from build123d import *

# Parameters (mm, degrees)
SKETCH1_W           = 44.45
SKETCH1_H           = 19.05
SKETCH1_W_2         = 38.1
SKETCH1_H_2         = 12.7
BOSS_EXTRUDE1_DEPTH = 12.7
CUT_EXTRUDE1_REACH  = 33.908
SKETCH2_R           = 2.0955
SKETCH3_W           = 50.8
SKETCH3_H           = 25.4
BOSS_EXTRUDE2_DEPTH = 3.175


with BuildPart() as part:
    # Sketch1 → Boss-Extrude1 (new body)
    with BuildSketch(Plane.XY):
        Rectangle(SKETCH1_W, SKETCH1_H)
        Rectangle(SKETCH1_W_2, SKETCH1_H_2, mode=Mode.SUBTRACT)
    extrude(amount=BOSS_EXTRUDE1_DEPTH)

    # Cut-Extrude1: up to this face of the body (flat: up to its plane)
    cut_extrude1_end = Plane(part.part.faces().sort_by_distance((0, -9.525, 6.35))[0])
    # Sketch2 → Cut-Extrude1 (cut, up to the picked face)
    with BuildSketch(Plane(origin=(0, 9.525, 0), x_dir=(1, 0, 0), z_dir=(0, 1, 0)), mode=Mode.PRIVATE) as cut_extrude1_sk1:
        with Locations(Location((-12.7, -6.35, 0), (0, 0, 270))):
            Circle(SKETCH2_R)
    cut_extrude1_tool1 = split(extrude(cut_extrude1_sk1.sketch, amount=-CUT_EXTRUDE1_REACH, mode=Mode.PRIVATE), bisect_by=cut_extrude1_end, keep=Keep.BOTH, mode=Mode.PRIVATE)
    # Sketch2 → Cut-Extrude1 (cut, up to the picked face)
    with BuildSketch(Plane(origin=(0, 9.525, 0), x_dir=(1, 0, 0), z_dir=(0, 1, 0)), mode=Mode.PRIVATE) as cut_extrude1_sk2:
        with Locations(Location((12.7, -6.35, 0), (0, 0, 90))):
            Circle(SKETCH2_R)
    cut_extrude1_tool2 = split(extrude(cut_extrude1_sk2.sketch, amount=-CUT_EXTRUDE1_REACH, mode=Mode.PRIVATE), bisect_by=cut_extrude1_end, keep=Keep.BOTH, mode=Mode.PRIVATE)
    add(cut_extrude1_tool1.solids().sort_by(Axis((-12.7, 9.525, 6.35), (0, -1, 0)))[0], mode=Mode.SUBTRACT)
    add(cut_extrude1_tool2.solids().sort_by(Axis((12.7, 9.525, 6.35), (0, -1, 0)))[0], mode=Mode.SUBTRACT)

    # Sketch3 → Boss-Extrude2 (add)
    with BuildSketch(Plane(origin=(0, 0, 0), x_dir=(-1, 0, 0), z_dir=(0, 0, -1))):
        Rectangle(SKETCH3_W, SKETCH3_H)
    extrude(amount=BOSS_EXTRUDE2_DEPTH)


solid = part.part
Build history of the part. All positions in model axes, mm. A direction names the side the tool comes from. Coordinates: 2 decimals unless noted, no trailing zeros. Write each loop counter-clockwise with the first axis right and the second up, starting at its lowest first coordinate (ties: lowest second). Pieces come first, ordered by that corner, then holes.
(1) Cut at A-A on x = 12.7. State how many separate pieces and enclosed holes the cut face has, and give its area (3 significant figures).
(2) Mould opens along Z. For faces 4 (the flat face through (-0.3, 6.5, 12.7)), 5 (the cylindrical face through (-10.62, -7.92, 6.08)), 6 (the flat face through (0, 0, -3.175)) say: pulls with the +Z half, pulls with the -Z half, needs draft (parallel to the pull), parting line crosses it, or undercut.
(3) Cut at D-D on x = -7. List the corners of the cut face in (y, z) (3 decimals), and give its area (3 significant figures).
(4) Cut at C-C on y = 2.5. List the corners of the cut face in (x, z) (3 decimals), and give its area (3 significant figures).
(5) Drill centre lines: line 1 (X direction, y = -7.8, z = 6.35) (1 decimal); line 2 (X direction, y = -4.25, z = 7.5) (3 decimals); line 3 (Y direction, x = 18.5, z = 2) (3 decimals). Where is each one in solid material? Low to high.
(6) Pin check, flat tips, straight feed: pin 1 Ø3.5 at (x, z) = (12.7, 6.35) entering from +Y; pin 2 Ø2 at (y, z) = (-3.5, 3) entering from +X (3 decimals); pin 3 Ø4 at (x, z) = (5, 6) entering from -Y (3 decimals); pin 4 Ø3 at (x, z) = (-18, 11) entering from +Y (3 decimals). Stop position of each tip, or through.
(7) 3-axis set-ups, long thin cutter, end or side, ignore diameter. For faces 1 (the flat face through (0, 9.525, 6)), 2 (the flat face through (19.05, 0, 6)), 3 (the flat face through (-22.225, 0, 6)): which of +Z, -Z, +X, -X, +Y, -Y reach the whole face in a straight line?
Working result:
1. separate pieces: 3
1. enclosed holes: 0
1. area: 135 mm2
2. face 4: pulls with the +Z half
2. face 5: undercut
2. face 6: pulls with the -Z half
3. outline: (-12.7, -3.175) - (12.7, -3.175) - (12.7, 0) - (9.525, 0) - (9.525, 12.7) - (6.35, 12.7) - (6.35, 0) - (-6.35, 0) - (-6.35, 12.7) - (-9.525, 12.7) - (-9.525, 0) - (-12.7, 0) - close
3. area: 161 mm2
4. outline: (-25.4, -3.175) - (25.4, -3.175) - (25.4, 0) - (22.225, 0) - (22.225, 12.7) - (19.05, 12.7) - (19.05, 0) - (-19.05, 0) - (-19.05, 12.7) - (-22.225, 12.7) - (-22.225, 0) - (-25.4, 0) - close
4. area: 242 mm2
5. line 1: x = -22.2 to -14.8, -10.6 to 10.6, 14.8 to 22.2
5. line 2: x = -22.225 to -19.05, 19.05 to 22.225
5. line 3: y = -9.525 to -6.35, 6.35 to 9.525
6. pin 1: passes through
6. pin 2: stops at x = 22.225
6. pin 3: stops at y = -9.525
6. pin 4: stops at y = 9.525
7. face 1: +Z, +X, -X, +Y
7. face 2: +Z
7. face 3: +Z, -X, +Y, -Y
